```python
from build123d import *

# Parameters (mm, degrees)
SKETCH1_W                       = 30
SKETCH1_H                       = 17
BOSS_EXTRUDE1_DEPTH             = 1.2446
M1_6_CLEARANCE_HOLE1_AT_2_COUNT = 2
M1_6_CLEARANCE_HOLE1_AT_2_PITCH = 16
M1_6_CLEARANCE_HOLE1_AT_3_COUNT = 2
M1_6_CLEARANCE_HOLE1_AT_3_PITCH = 13.4
M1_6_CLEARANCE_HOLE1_AT_4_COUNT = 2
M1_6_CLEARANCE_HOLE1_AT_4_PITCH = 20.870074269
F_2_CLEARANCE_HOLE1_D           = 2.2606
F_2_CLEARANCE_HOLE1_DEPTH       = 2.032
F_2_CLEARANCE_HOLE1_TIP         = 0.679152758


with BuildPart() as part:
    # Sketch1 → Boss-Extrude1 (new body)
    with BuildSketch(Plane(origin=(0, 0, 0), x_dir=(1, 0, 0), z_dir=(0, 1, 0))):
        Rectangle(SKETCH1_W, SKETCH1_H)
    extrude(amount=BOSS_EXTRUDE1_DEPTH)

    # Sketch4 → M1.6 Clearance Hole1 (revolve, cut)
    with BuildSketch(Plane(origin=(-8, 0, 6.407104521), x_dir=(0, 0, -1), z_dir=(1, 0, 0))):
        Polygon((0, 0), (0, 1.2446), (0.9, 1.2446), (0.9, 0.6), (1.5, 0), align=None)
    m1_6_clearance_hole1 = revolve(axis=Axis((-8, -6.35, 6.407104521), (0, 1, 0)), mode=Mode.SUBTRACT)

    # M1.6 Clearance Hole1 at 2: M1.6 Clearance Hole1 ×2
    with Locations(*[(i * M1_6_CLEARANCE_HOLE1_AT_2_PITCH, 0, 0) for i in range(1, M1_6_CLEARANCE_HOLE1_AT_2_COUNT)]):
        add(m1_6_clearance_hole1, mode=Mode.SUBTRACT)

    # M1.6 Clearance Hole1 at 3: M1.6 Clearance Hole1 ×2
    with Locations(*[(0, 0, -i * M1_6_CLEARANCE_HOLE1_AT_3_PITCH) for i in range(1, M1_6_CLEARANCE_HOLE1_AT_3_COUNT)]):
        add(m1_6_clearance_hole1, mode=Mode.SUBTRACT)

    # M1.6 Clearance Hole1 at 4: M1.6 Clearance Hole1 ×2
    with Locations(*[Vector(0.766647967, 0, -0.642067672) * (i * M1_6_CLEARANCE_HOLE1_AT_4_PITCH) for i in range(1, M1_6_CLEARANCE_HOLE1_AT_4_COUNT)]):
        add(m1_6_clearance_hole1, mode=Mode.SUBTRACT)

    # #2 Clearance Hole1
    with Locations(Plane(origin=(0, 1.2446, 0), x_dir=(-1, 0, 0), z_dir=(0, 1, 0))):
        with Locations((13, -6.5), (13, 6.5), (-13, -6.5), (-13, 6.5)):
            Hole(F_2_CLEARANCE_HOLE1_D / 2, depth=F_2_CLEARANCE_HOLE1_DEPTH)
            with Locations((0, 0, -(F_2_CLEARANCE_HOLE1_DEPTH + F_2_CLEARANCE_HOLE1_TIP / 2))):  # 118° drill point
                Cone(0, F_2_CLEARANCE_HOLE1_D / 2, F_2_CLEARANCE_HOLE1_TIP, mode=Mode.SUBTRACT)


solid = part.part
```
Can you work these out from the model? Positions are in its coordinate system, mm. Coordinates: 2 decimals unless noted, no trailing zeros. Order: outer loops, then holes, each group sorted by start corner. A loop starts at its lowest first (then second) coordinate and runs counter-clockwise, first axis right, second up. Notation, with made-up numbers: (64.5, 75) -> (102.5, 75) arc R28 cw to (102.5, 111) -> close; hole circle Ø3 at (69.25, -22). An arc over 180 degrees is marked (long way). Write each question's results on one line, items separated by ' | '.
Item 1: I want a section at B-B, the plane y = 1. Count the separate pieces of the cut face and the enclosed holes in it, then the cut area to 3 significant figures.
Results are:
separate pieces: 1 | enclosed holes: 8 | area: 484 mm²
Item 2: I want a section at A-A, the plane x = 13. Write out the boundary of the cut face in (y, z).
Results are:
outline: (0, -8.5) -> (1.24, -8.5) -> (1.24, -7.63) -> (0, -7.63) -> close; (0, -5.37) -> (1.24, -5.37) -> (1.24, 5.37) -> (0, 5.37) -> close; (0, 7.63) -> (1.24, 7.63) -> (1.24, 8.5) -> (0, 8.5) -> close
Item 3: If we mould it in two halves opening along Z, with no side actions, what happens to faces 1 (the face through (0, 1, -8.5)), 2 (the face through (-13.897, 0.614, -7.188)), 3 (the face through (15, 1, 0))? For each: +Z half, -Z half, draft (parallel to the pull), parting line (faces both ways), or undercut.
Results are:
face 1: -Z half | face 2: undercut | face 3: draft
Item 4: If I drill on line 1 along Z through (x, y) = (-8, 1.05); line 2 along Z through (x, y) = (-13, 0.65); line 3 along X through (y, z) = (0.3, 7), over which ranges is the centre line in solid material (lowest first)?
Results are:
line 1: -8.5 to -7.89, -6.09 to 5.51, 7.31 to 8.5 | line 2: -8.5 to -7.63, -5.37 to 5.37, 7.63 to 8.5 | line 3: -15 to -14.01, -11.99 to -9.04, -6.96 to 6.96, 9.04 to 11.99, 14.01 to 15
Item 5: I'm going to push a flat-ended pin straight in: pin 1 Ø2.5 at (x, z) = (-8, -6.99) entering from -Y. Where does the tip first touch, or does it pass through?
Results are:
pin 1: y = 0.25
